from build123d import *

# Parameters (mm, degrees)
SKETCH1_W           = 58
SKETCH1_H           = 48
BOSS_EXTRUDE1_DEPTH = 5
SKETCH2_R           = 2
SKETCH2_R_2         = 1.5
CUT_EXTRUDE1_DEPTH  = 5
FILLET1_R           = 5
FILLET2_R           = 5
FILLET3_R           = 5
FILLET4_R           = 5


with BuildPart() as part:
    # Sketch1 → Boss-Extrude1 (new body)
    with BuildSketch(Plane(origin=(0, 0, 0), x_dir=(1, 0, 0), z_dir=(0, 1, 0))):
        Rectangle(SKETCH1_W, SKETCH1_H)
    extrude(amount=BOSS_EXTRUDE1_DEPTH)

    # Sketch2 → Cut-Extrude1 (cut)
    with BuildSketch(Plane(origin=(0, 5, 0), x_dir=(1, 0, 0), z_dir=(0, 1, 0))):
        with Locations((21, -16)):
            Circle(SKETCH2_R)
        with Locations((-21, -16)):
            Circle(SKETCH2_R)
        with Locations((-21, 16)):
            Circle(SKETCH2_R)
        with Locations((21, 16)):
            Circle(SKETCH2_R)
        with Locations((9.5, -9.5)):
            Circle(SKETCH2_R_2)
        with Locations((-9.5, -9.5)):
            Circle(SKETCH2_R_2)
        with Locations((9.5, 9.5)):
            Circle(SKETCH2_R_2)
        with Locations((-9.5, 9.5)):
            Circle(SKETCH2_R_2)
    extrude(amount=-CUT_EXTRUDE1_DEPTH, mode=Mode.SUBTRACT)

    # Fillet1
    fillet1_edges = [part.edges().sort_by_distance(p)[0] for p in [
        (-29, 2.5, 24),
    ]]
    fillet(fillet1_edges, radius=FILLET1_R)

    # Fillet2
    fillet2_edges = [part.edges().sort_by_distance(p)[0] for p in [
        (29, 2.5, 24),
    ]]
    fillet(fillet2_edges, radius=FILLET2_R)

    # Fillet3
    fillet3_edges = [part.edges().sort_by_distance(p)[0] for p in [
        (29, 2.5, -24),
    ]]
    fillet(fillet3_edges, radius=FILLET3_R)

    # Fillet4
    fillet4_edges = [part.edges().sort_by_distance(p)[0] for p in [
        (-29, 2.5, -24),
    ]]
    fillet(fillet4_edges, radius=FILLET4_R)


solid = part.part
Model file for the job. Use its own axes, mm. Give positions to 0.01 mm unless a question says otherwise; leave off trailing zeros. Write each loop counter-clockwise with the first axis right and the second up, starting at its lowest first coordinate (ties: lowest second). Pieces come first, ordered by that corner, then holes. Notation, with made-up numbers: M 41.5,40 L 91.5,40 A30 ccw 91.5,71 Z; hole C 55,-18 d1. An arc over 180 degrees is marked long. One line per item, written item: value. Start each with the question number.
Q1. Saw through at A-A, the plane z = -16. Write the cut outline in (x, y), plus the area to 3 significant figures.
Q2. Two-plate mould, pull along X, no slides. Class faces 1 (the cylindrical face through (-21, 3, -18)), 2 (the flat face through (0, 5, 0)), 3 (the cylindrical face through (28, 3, -22)): +X half, -X half, draft (parallel to the pull), parting line (faces both ways), or undercut.
Q3. Probe probe 1 along X at (y, z) = (3.95, -9.5); probe 2 along Z at (x, y) = (21, 2.15); probe 3 along Z at (x, y) = (-9.5, 1.3). List the from-to ranges inside material, lowest first. Write a range as [from, to].
Q4. Saw through at C-C, the plane y = 3.9. State how many separate pieces and enclosed holes the cut face has, plus the area to 3 significant figures.
Q5. Saw through at B-B, the plane x = -9.5. Write the cut outline in (y, z).
Output values:
1. outline: M -29,0 L -23,0 L -23,5 L -29,5 Z; M -19,0 L 19,0 L 19,5 L -19,5 Z; M 23,0 L 29,0 L 29,5 L 23,5 Z
1. area: 250 mm²
2. face 1: undercut
2. face 2: draft
2. face 3: +X half
3. probe 1: x = [-29, -11], [-8, 8], [11, 29]
3. probe 2: z = [-24, -18], [-14, 14], [18, 24]
3. probe 3: z = [-24, -11], [-8, 8], [11, 24]
4. separate pieces: 1
4. enclosed holes: 8
4. area: 2,680 mm²
5. outline: M 0,-24 L 5,-24 L 5,-11 L 0,-11 Z; M 0,-8 L 5,-8 L 5,8 L 0,8 Z; M 0,11 L 5,11 L 5,24 L 0,24 Z
